```python
from build123d import *

# Parameters (mm, degrees)
SKETCH_1_W             = 55
SKETCH_1_H             = 40
EXTRUDE_1_DEPTH        = 4
CUT_EXTRUDE_START      = 4
SKETCH_1_6_OUTSIDE_W   = 70.624
SKETCH_1_6_OUTSIDE_H   = 55.624
SKETCH_1_6_OUTSIDE_W_2 = 55
SKETCH_1_6_OUTSIDE_H_2 = 40
SKETCH_1_6_OUTSIDE_R   = 4
SKETCH_1_6_OUTSIDE_R_2 = 1.5
CUT_EXTRUDE_5_DEPTH    = 5
FILLET_4_R             = 4
FILLET_6_R             = 4
FILLET_7_R             = 4
FILLET_8_R             = 4
SKETCH_2_R             = 9.705576387
EXTRUDE_2_DEPTH        = 3
CUT_EXTRUDE_START_2    = -5
CUT_EXTRUDE_7_DEPTH    = 5
SKETCH_4_R             = 0.44
CUT_EXTRUDE_8_DEPTH    = 2


with BuildPart() as part:
    # 草图1 → 凸台-拉伸1 (new body)
    with BuildSketch(Plane(origin=(0, 0, 0), x_dir=(1, 0, 0), z_dir=(0, 1, 0))):
        Rectangle(SKETCH_1_W, SKETCH_1_H)
    extrude(amount=EXTRUDE_1_DEPTH)

    # 草图1<6> outside → 切除-拉伸5 (cut)
    # profile 1 of 6: a face of its own
    with BuildSketch(Plane(origin=(0, 0, 0), x_dir=(1, 0, 0), z_dir=(0, 1, 0)).offset(CUT_EXTRUDE_START)):
        Rectangle(SKETCH_1_6_OUTSIDE_W, SKETCH_1_6_OUTSIDE_H)
        Rectangle(SKETCH_1_6_OUTSIDE_W_2, SKETCH_1_6_OUTSIDE_H_2, mode=Mode.SUBTRACT)
    # profile 2 of 6: a face of its own
    with BuildSketch(Plane(origin=(0, 0, 0), x_dir=(1, 0, 0), z_dir=(0, 1, 0)).offset(CUT_EXTRUDE_START)):
        with Locations(Location((0, 0, 0), (0, 0, 270))):
            Circle(SKETCH_1_6_OUTSIDE_R)
    # profile 3 of 6: a face of its own
    with BuildSketch(Plane(origin=(0, 0, 0), x_dir=(1, 0, 0), z_dir=(0, 1, 0)).offset(CUT_EXTRUDE_START)):
        with Locations(Location((-17.5, 14, 0), (0, 0, 270))):
            Circle(SKETCH_1_6_OUTSIDE_R_2)
    # profile 4 of 6: a face of its own
    with BuildSketch(Plane(origin=(0, 0, 0), x_dir=(1, 0, 0), z_dir=(0, 1, 0)).offset(CUT_EXTRUDE_START)):
        with Locations(Location((17.5, 14, 0), (0, 0, 270))):
            Circle(SKETCH_1_6_OUTSIDE_R_2)
    # profile 5 of 6: a face of its own
    with BuildSketch(Plane(origin=(0, 0, 0), x_dir=(1, 0, 0), z_dir=(0, 1, 0)).offset(CUT_EXTRUDE_START)):
        with Locations(Location((17.5, -14, 0), (0, 0, 270))):
            Circle(SKETCH_1_6_OUTSIDE_R_2)
    # profile 6 of 6: a face of its own
    with BuildSketch(Plane(origin=(0, 0, 0), x_dir=(1, 0, 0), z_dir=(0, 1, 0)).offset(CUT_EXTRUDE_START)):
        with Locations(Location((-17.5, -14, 0), (0, 0, 270))):
            Circle(SKETCH_1_6_OUTSIDE_R_2)
    extrude(amount=-CUT_EXTRUDE_5_DEPTH, mode=Mode.SUBTRACT)

    # 圆角4
    fillet_4_edges = [part.edges().sort_by_distance(p)[0] for p in [
        (27.5, 0, 0),
    ]]
    fillet(fillet_4_edges, radius=FILLET_4_R - 0.0001)  # a hair under: the kernel refuses the full size

    # 圆角6
    fillet_6_edges = [part.edges().sort_by_distance(p)[0] for p in [
        (26.328456414, 1.171543586, 20),
        (-1.99995, 0, 20),
    ]]
    fillet(fillet_6_edges, radius=FILLET_6_R - 0.0001)  # a hair under: the kernel refuses the full size

    # 圆角7
    fillet_7_edges = [part.edges().sort_by_distance(p)[0] for p in [
        (-27.5, 1.171543586, 18.828456414),
        (-27.5, 0, -1.99995),
    ]]
    fillet(fillet_7_edges, radius=FILLET_7_R - 0.0001)  # a hair under: the kernel refuses the full size

    # 圆角8
    fillet_8_edges = [part.edges().sort_by_distance(p)[0] for p in [
        (26.328456414, 1.171543586, -20),
        (0, 0, -20),
        (-26.328456414, 1.171543586, -20),
    ]]
    fillet(fillet_8_edges, radius=FILLET_8_R - 0.0001)  # a hair under: the kernel refuses the full size

    # 草图2 → 凸台-拉伸2 (add)
    with BuildSketch(Plane.XZ):
        with Locations(Location((0, 0, 0), (0, 0, 90))):
            Circle(SKETCH_2_R)
    extrude(amount=EXTRUDE_2_DEPTH)

    # 草图3 → 切除-拉伸7 (cut)
    with BuildSketch(Plane(origin=(0, -3, 0), x_dir=(-1, 0, 0), z_dir=(0, -1, 0)).offset(CUT_EXTRUDE_START_2)):
        with BuildLine():
            Line((3.226722166, -9.153495347), (4.917462581, 0))
            Line((4.917462581, 0), (3.226722166, 9.153495347))
            ThreePointArc((3.226722166, 9.153495347), (0, 9.705576387), (-3.226722166, 9.153495347))
            Line((-3.226722166, 9.153495347), (-4.917462581, 0))
            Line((-4.917462581, 0), (-3.226722166, -9.153495347))
            ThreePointArc((-3.226722166, -9.153495347), (0, -9.705576387), (3.226722166, -9.153495347))
        make_face()
    extrude(amount=CUT_EXTRUDE_7_DEPTH, mode=Mode.SUBTRACT)

    # 草图4 → 切除-拉伸8 (cut)
    with BuildSketch(Plane.XZ):
        with Locations(Location((0.243749782, -11.478919209, 0), (0, 0, 270))):
            Circle(SKETCH_4_R)
    extrude(amount=-CUT_EXTRUDE_8_DEPTH, mode=Mode.SUBTRACT)


solid = part.part
```
Could you check a few things on this model? Use its own coordinates, in mm. A direction names the side the tool comes from. Coordinates: 2 decimals unless noted, no trailing zeros. Order: outer loops, then holes, each group sorted by start corner. A loop starts at its lowest first (then second) coordinate and runs counter-clockwise, first axis right, second up. Notation, with made-up numbers: M 65.5,-33 L 124.5,-33 A22 cw 124.5,3 Z; hole C -33,73 d10. An arc over 180 degrees is marked long. Use one line per item in the form item = value. Start each with the question number.
1. Please list where these lines run through material, in increasing order: line 1 (X direction, y = 2.4, z = -14); line 2 (X direction, y = 1.8, z = 14); line 3 (Y direction, x = 15, z = 13.5).
2. For pin 1 (5 mm diameter, centred on x = 1, z = -13, fed in from -Y); pin 2 (7 mm diameter, centred on x = 0, z = 0, fed in from -Y); pin 3 (1.5 mm diameter, centred on x = 12.5, y = 0.5, fed in from -Z); pin 4 (2 mm diameter, centred on y = 1, z = 2.5, fed in from -X), each with a flat end and sliding along its axis, tell me the tip position at first contact or that it passes through.
3. Suppose I cut it at B-B on y = -2.25. Write out the boundary of the cut face in (x, z), then the cut area to 3 significant figures.
4. We'd pull the mould along X, two halves only. Please class faces 5 (the cylindrical face through (26.297, 1.141, -0.224)), 6 (the flat face through (4.06, -0.46, -4.64)), 7 (the flat face through (10, 0, 0)), 8 (the flat face through (4.084, -0.465, 4.513)): +X half, -X half, draft (parallel to the pull), parting line (faces both ways), or undercut.
5. Suppose I cut it at A-A on x = 17.5. Count the separate pieces of the cut face and the enclosed holes in it, then the cut area to 3 significant figures.
6. On a 3-axis mill with a long thin cutter (end or side, diameter ignored), from which of +Z, -Z, +X, -X, +Y, -Y can I reach the whole of each face in a straight line? I mean faces 1 (the cylindrical face through (9.704, -1.479, -0.167)), 2 (the cylindrical face through (-9.704, -1.479, 0.167)), 3 (the cylindrical face through (0.329, 1.203, 18.859)), 4 (the flat face through (0.1, 2, 4.2)). Say none if no direction works.
Geometry says:
q1.line_1 = -27.17 to -19, -16 to 16, 19 to 27.17
q1.line_2 = -26.84 to -19, -16 to 16, 19 to 26.84
q1.line_3 = 0 to 4
q2.pin_1 = 0
q2.pin_2 = through
q2.pin_3 = -18.9
q2.pin_4 = -26.96
q3.outline = M -4.92,0 L -3.23,9.15 A9.71 ccw -3.23,-9.15 Z; M 3.23,-9.15 A9.71 ccw 3.23,9.15 L 4.92,0 Z
q3.area = 142 mm^2
q4.face_5 = +X half
q4.face_6 = undercut
q4.face_7 = draft
q4.face_8 = undercut
q5.separate_pieces = 3
q5.enclosed_holes = 0
q5.area = 129 mm^2
q6.face_1 = +X, -Y
q6.face_2 = -X, -Y
q6.face_3 = +Z, +X, -X, -Y
q6.face_4 = -Y
